Answer from the drawing. Dimensions are ordinates in mm from the lowest x, y and z of the part. A direction names the side the tool comes from. Give positions to 0.01 mm unless a question says otherwise; leave off trailing zeros. Loops run counter-clockwise (first coordinate to the right, second up) from the corner with the lowest first, then second, coordinate; pieces in that order, holes last. Notation, with made-up numbers: (17.5, 75) - (34.5, 75) arc R14 cw to (34.5, 83) - close; hole circle Ø6 at (-31.75, 88.5). An arc over 180 degrees is marked (long way). Put each result on its own line as item: value. Start each with the question number.
1. A cutting plane is placed at A-A, the plane x = 35. Determine the outline of the cut face in (y, z).
2. For a pull along X with two mould halves and no side action, classify the marked faces 1, 2, 3 and 4 as released by +X, released by -X, zero draft, split by the parting line, or undercut.
3. A cutting plane is placed at D-D, the plane x = 62.5. Determine the outline of the cut face in (y, z), plus the area to 3 significant figures.
4. A cutting plane is placed at C-C, the plane y = 21.5. Determine the outline of the cut face in (x, z).
5. Given pin 1 Ø10 at (x, y) = (63, 29.5) entering from -Z; pin 2 Ø15 at (y, z) = (8.5, 39) entering from -X; pin 3 Ø3 at (y, z) = (28.5, 6) entering from +X; pin 4 Ø13 at (x, z) = (35, 45) entering from +Y, each flat-ended and moving along its own axis, determine where each tip first touches the part or whether it passes through.
6. For the marked faces 5, 6, 7, 8 and 9, determine the directions among +Z, -Z, +X, -X, +Y, -Y from which every point of the face is accessible in a straight line to the end or side of a thin tool.
7. A cutting plane is placed at B-B, the plane z = 45. Determine the outline of the cut face in (x, y).
8. Consider L1, parallel to Z at x = 35, y = 26.25; L2, parallel to Z at x = 35, y = 33.75; L3, parallel to Y at x = 42.5, z = 41. Determine where each line is inside the solid, lowest interval first. Write a range as from..to.
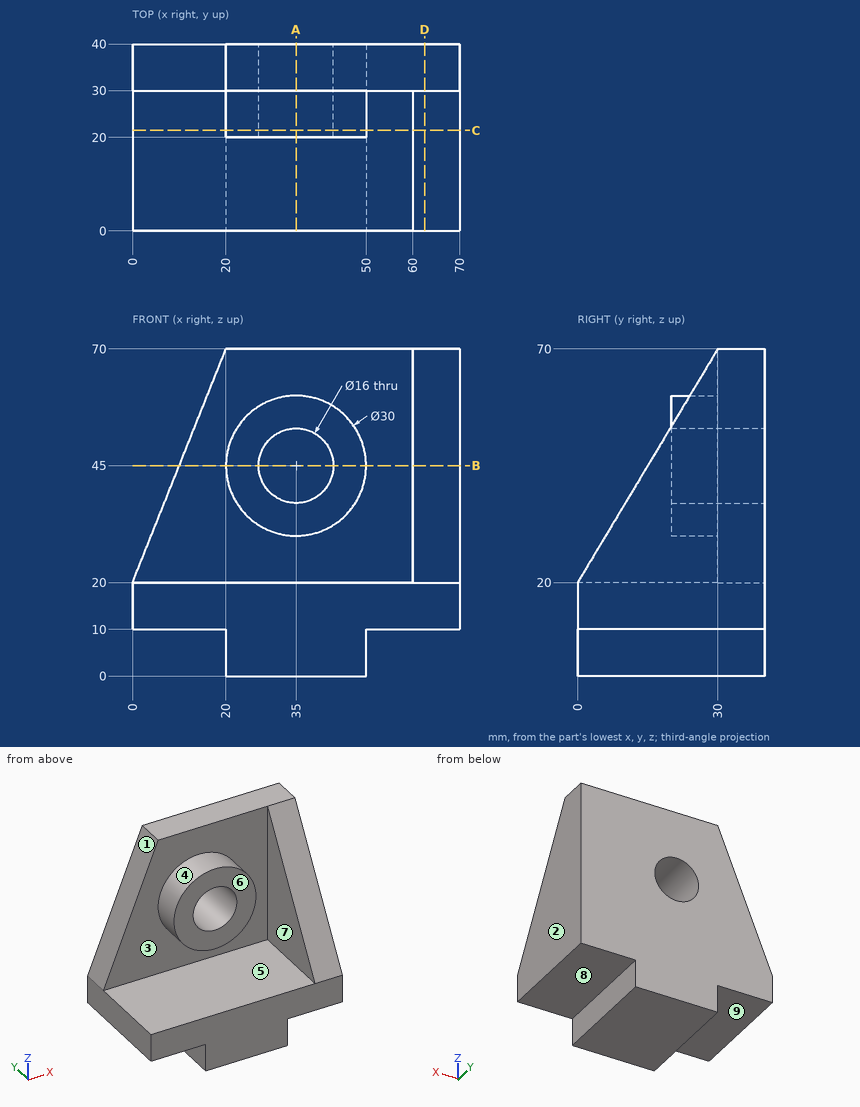
Return value:
1. outline: (0, 0) - (40, 0) - (40, 37) - (20, 37) - (20, 30) - (30, 30) - (30, 20) - (0, 20) - close; (20, 53) - (40, 53) - (40, 70) - (30, 70) - (30, 60) - (20, 60) - close
2. face 1: released by -X
2. face 2: released by +X
2. face 3: undercut
2. face 4: undercut
3. outline: (0, 10) - (40, 10) - (40, 70) - (30, 70) - (0, 20) - close
3. area: 1,650 mm2
4. outline: (0, 10) - (20, 10) - (20, 0) - (50, 0) - (50, 10) - (70, 10) - (70, 55.83) - (60, 55.83) - (60, 20) - (0, 20) - close; circle Ø30 at (35, 45); hole circle Ø16 at (35, 45)
5. pin 1: stops at z = 10
5. pin 2: stops at x = 60
5. pin 3: stops at x = 50
5. pin 4: passes through
6. face 5: -X, -Y
6. face 6: +Z, -X, -Y
6. face 7: +Z, -Y
6. face 8: -Z, +X, +Y, -Y
6. face 9: -Z, -X, +Y, -Y
7. outline: (10, 30) - (20, 30) - (20, 20) - (27, 20) - (27, 40) - (10, 40) - close; (43, 20) - (50, 20) - (50, 30) - (60, 30) - (60, 15) - (70, 15) - (70, 40) - (43, 40) - close
8. L1: z = 0..20, 30..37, 53..60
8. L2: z = 0..37, 53..70
8. L3: y = 20..40
